Read the model definition and answer for the solid it produces. Units are mm, in the model's axes. Coordinates: 2 decimals unless noted, no trailing zeros.
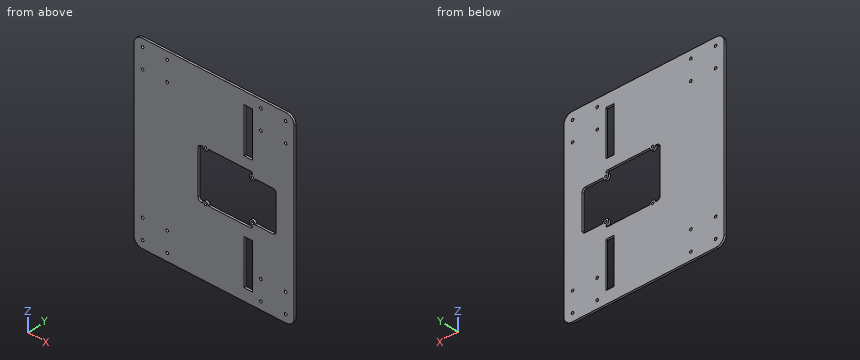
from build123d import *

# Parameters (mm, degrees)
SKETCH_1_W          = 51
SKETCH_1_H          = 44
SKETCH_1_R          = 1.6
SKETCH_1_W_2        = 10
SKETCH_1_H_2        = 15
EXTRUDE_1_DEPTH     = 2.5
SKETCH_2_R          = 1.5
CUT_EXTRUDE_1_DEPTH = 2.5
FILLET_1_R          = 10
FILLET_2_R          = 4
FILLET_3_R          = 2


with BuildPart() as part:
    # 草图1 → 凸台-拉伸1 (new body)
    # profile 1 of 7: a face of its own
    with BuildSketch(Plane(origin=(0, 0, 0), x_dir=(1, 0, 0), z_dir=(0, 1, 0))):
        Polygon((134, 0), (134, 15), (134, 71), (144, 71), (144, 44), (195, 44), (195, 186), (144, 186), (144, 159), (134, 159), (134, 215), (134, 230), (51, 230), (51, 186), (0, 186), (0, 44), (51, 44), (51, 0), align=None)
    # profile 2 of 7: a face of its own
    with BuildSketch(Plane(origin=(0, 0, 0), x_dir=(1, 0, 0), z_dir=(0, 1, 0))):
        with Locations((25.5, 208)):
            Rectangle(SKETCH_1_W, SKETCH_1_H)
        with Locations(Location((10.5, 196, 0), (0, 0, 270))):
            Circle(SKETCH_1_R, mode=Mode.SUBTRACT)
        with Locations(Location((40.5, 196, 0), (0, 0, 270))):
            Circle(SKETCH_1_R, mode=Mode.SUBTRACT)
        with Locations(Location((10.5, 220.5, 0), (0, 0, 270))):
            Circle(SKETCH_1_R, mode=Mode.SUBTRACT)
        with Locations(Location((40.5, 220.5, 0), (0, 0, 270))):
            Circle(SKETCH_1_R, mode=Mode.SUBTRACT)
    # profile 3 of 7: a face of its own
    with BuildSketch(Plane(origin=(0, 0, 0), x_dir=(1, 0, 0), z_dir=(0, 1, 0))):
        Polygon((144, 186), (195, 186), (195, 230), (144, 230), (144, 215), align=None)
        with Locations(Location((154.5, 196, 0), (0, 0, 270))):
            Circle(SKETCH_1_R, mode=Mode.SUBTRACT)
        with Locations(Location((184.5, 196, 0), (0, 0, 270))):
            Circle(SKETCH_1_R, mode=Mode.SUBTRACT)
        with Locations(Location((154.5, 220.5, 0), (0, 0, 270))):
            Circle(SKETCH_1_R, mode=Mode.SUBTRACT)
        with Locations(Location((184.5, 220.5, 0), (0, 0, 270))):
            Circle(SKETCH_1_R, mode=Mode.SUBTRACT)
    # profile 4 of 7: a face of its own
    with BuildSketch(Plane(origin=(0, 0, 0), x_dir=(1, 0, 0), z_dir=(0, 1, 0))):
        with Locations((25.5, 22)):
            Rectangle(SKETCH_1_W, SKETCH_1_H)
        with Locations(Location((10.5, 9.5, 0), (0, 0, 270))):
            Circle(SKETCH_1_R, mode=Mode.SUBTRACT)
        with Locations(Location((40.5, 9.5, 0), (0, 0, 270))):
            Circle(SKETCH_1_R, mode=Mode.SUBTRACT)
        with Locations(Location((10.5, 34, 0), (0, 0, 270))):
            Circle(SKETCH_1_R, mode=Mode.SUBTRACT)
        with Locations(Location((40.5, 34, 0), (0, 0, 270))):
            Circle(SKETCH_1_R, mode=Mode.SUBTRACT)
    # profile 5 of 7: a face of its own
    with BuildSketch(Plane(origin=(0, 0, 0), x_dir=(1, 0, 0), z_dir=(0, 1, 0))):
        Polygon((144, 44), (144, 15), (144, 0), (195, 0), (195, 44), align=None)
        with Locations(Location((154.5, 9.5, 0), (0, 0, 270))):
            Circle(SKETCH_1_R, mode=Mode.SUBTRACT)
        with Locations(Location((184.5, 9.5, 0), (0, 0, 270))):
            Circle(SKETCH_1_R, mode=Mode.SUBTRACT)
        with Locations(Location((154.5, 34, 0), (0, 0, 270))):
            Circle(SKETCH_1_R, mode=Mode.SUBTRACT)
        with Locations(Location((184.5, 34, 0), (0, 0, 270))):
            Circle(SKETCH_1_R, mode=Mode.SUBTRACT)
    # profile 6 of 7: a face of its own
    with BuildSketch(Plane(origin=(0, 0, 0), x_dir=(1, 0, 0), z_dir=(0, 1, 0))):
        with Locations((139, 7.5)):
            Rectangle(SKETCH_1_W_2, SKETCH_1_H_2)
    # profile 7 of 7: a face of its own
    with BuildSketch(Plane(origin=(0, 0, 0), x_dir=(1, 0, 0), z_dir=(0, 1, 0))):
        with Locations((139, 222.5)):
            Rectangle(SKETCH_1_W_2, SKETCH_1_H_2)
    extrude(amount=EXTRUDE_1_DEPTH)

    # 草图2 → 切除-拉伸1 (cut)
    with BuildSketch(Plane(origin=(0, 2.5, 0), x_dir=(1, 0, 0), z_dir=(0, 1, 0))):
        with Locations(Location((87, 84, 0), (0, 0, 270))):
            Circle(SKETCH_2_R)
        with BuildLine():
            ThreePointArc((83.5, 84), (87, 87.5), (90.5, 84))
            Line((90.5, 84), (144, 84))
            Line((144, 84), (144, 86.5))
            ThreePointArc((144, 86.5), (141.525126266, 92.474873734), (147.5, 90))
            Line((147.5, 90), (173, 90))
            Line((173, 90), (173, 140))
            Line((173, 140), (147.5, 140))
            ThreePointArc((147.5, 140), (141.525126266, 137.525126266), (144, 143.5))
            Line((144, 143.5), (144, 146))
            Line((144, 146), (90.5, 146))
            ThreePointArc((90.5, 146), (87, 142.5), (83.5, 146))
            Line((83.5, 146), (78, 146))
            Line((78, 146), (78, 84))
            Line((78, 84), (83.5, 84))
        make_face()
        with Locations(Location((144, 90, 0), (0, 0, 270))):
            Circle(SKETCH_2_R)
        with Locations(Location((144, 140, 0), (0, 0, 270))):
            Circle(SKETCH_2_R)
        with Locations(Location((87, 146, 0), (0, 0, 270))):
            Circle(SKETCH_2_R)
    extrude(amount=-CUT_EXTRUDE_1_DEPTH, mode=Mode.SUBTRACT)

    # 圆角1
    fillet_1_edges = [part.edges().sort_by_distance(p)[0] for p in [
        (0, 1.25, 0),
        (0, 1.25, -230),
        (195, 1.25, -230),
        (195, 1.25, 0),
    ]]
    fillet(fillet_1_edges, radius=FILLET_1_R)

    # 圆角2
    fillet_2_edges = [part.edges().sort_by_distance(p)[0] for p in [
        (78, 1.25, -146),
        (78, 1.25, -84),
        (173, 1.25, -90),
        (173, 1.25, -140),
    ]]
    fillet(fillet_2_edges, radius=FILLET_2_R)

    # 圆角3
    fillet_3_edges = [part.edges().sort_by_distance(p)[0] for p in [
        (144, 1.25, -84),
        (144, 1.25, -146),
    ]]
    fillet(fillet_3_edges, radius=FILLET_3_R)


solid = part.part
Item 1: Given pin 1 (3 mm diameter, centred on x = 184.5, z = -9.5, fed in from -Y), flat-ended and moving along its own axis, determine where the tip first touches the part or whether it passes through.
Numbers:
pin 1: passes through
Item 2: Find the intervals of material crossed by line 1 along Z through (x, y) = (154.5, 1.45); line 2 along X through (y, z) = (0.9, -9.5); line 3 along X through (y, z) = (1.15, -196), in increasing order.
Numbers:
line 1: z = -230 to -222.1, -218.9 to -197.6, -194.4 to -140, -90 to -35.6, -32.4 to -11.1, -7.9 to 0
line 2: x = 0.01 to 8.9, 12.1 to 38.9, 42.1 to 152.9, 156.1 to 182.9, 186.1 to 194.99
line 3: x = 0 to 8.9, 12.1 to 38.9, 42.1 to 134, 144 to 152.9, 156.1 to 182.9, 186.1 to 195
Item 3: A cutting plane is placed at A-A on y = 0.8. Give the number of separate pieces and of enclosed holes in the cut face, then the cut area to 3 significant figures.
Numbers:
separate pieces: 1
enclosed holes: 23
area: 38,100 mm2
